Verification items for the finished model (mm, model axes). A direction names the side the tool comes from. Coordinates: 2 decimals unless noted, no trailing zeros. Order: outer loops, then holes, each group sorted by start corner. A loop starts at its lowest first (then second) coordinate and runs counter-clockwise, first axis right, second up. Notation, with made-up numbers: M -2,79 L 52,79 A32 ccw 52,109 Z; hole C 88,-1 d9. An arc over 180 degrees is marked long. Return JSON: item names as keys, results as strings.
Autodesk Inventor part; units mm, degrees
ref_plane "YZ Plane" through (0, 0, 0) normal (1, 0, 0) x (0, 1, 0)
ref_plane "XZ Plane" through (0, 0, 0) normal (0, 1, 0) x (-1, 0, 0)
ref_plane "XY Plane" through (0, 0, 0) normal (0, 0, 1) x (1, 0, 0)
sketch "Esquisse1" plane through (0, 0, 0) normal (0, 1, 0) x (-1, 0, 0)
  line L0 (28, -26) -> (-28, -26)
  line L1 (-28, -26) -> (-28, 26)
  line L2 (-28, 26) -> (28, 26)
  line L3 (28, 26) -> (28, -26)
  point P0 (0, 0)
  dimension "d0" = 56
  dimension "d1" = 28
  dimension "d2" = 52
  dimension "d3" = 26
extrude "Extrusion1" add sketch "Esquisse1" along normal blind 1.6
sketch "Esquisse2" plane through (0, 1.6, 0) normal (0, 1, 0) x (1, 0, 0)
  line L0 (-26, 24) -> (-23.5, 24)
  line L1 (-23.5, 24) -> (-23.5, -15)
  line L2 (-23.5, -15) -> (-26, -15)
  line L3 (-26, -15) -> (-26, 24)
  line L4 (22.5, 24) -> (25, 24)
  line L5 (25, 24) -> (25, -24)
  line L6 (25, -24) -> (22.5, -24)
  line L7 (22.5, -24) -> (22.5, 24)
  line L8 (28, 26) -> (-28, 26)
  line L9 (-28, 26) -> (-28, -26)
  point P0 (0, 0)
  dimension "d6" = 2.5
  dimension "d7" = 2.5
  dimension "d8" = 39
  dimension "d9" = 48
  dimension "d10" = 2
  dimension "d11" = 2
  dimension "d12" = 46
extrude "Extrusion2" add sketch "Esquisse2" along normal blind 3
properties part number "PCB Wifi" material "Nylon, disulfure de molybdène"
Q1. Draft check along X on faces 1 (the face through (-28, 1, 0)), 2 (the face through (22.5, 3, 0)), 3 (the face through (25, 3, 0)), 4 (the face through (-25, 3, 15)). Enter one of: pulls with the +X half, pulls with the -X half, needs draft (parallel to the pull), parting line crosses it, or undercut.
Values:
{"face 1": "pulls with the -X half", "face 2": "undercut", "face 3": "pulls with the +X half", "face 4": "needs draft"}
Q2. Tool access check on faces 5 (the face through (24, 3, -24)), 6 (the face through (24, 3, 24)), 7 (the face through (-23.5, 3, -5)), 8 (the face through (-26, 3, -4)). Record the directions out of +Z, -Z, +X, -X, +Y, -Y that give a thin tool (end or side, any length) a straight path to the whole face; none if there is none.
Values:
{"face 5": "-Z, +X, -X, +Y", "face 6": "+Z, +X, -X, +Y", "face 7": "+Z, -Z, +Y", "face 8": "+Z, -Z, -X, +Y"}
Q3. Cross-section at D-D, the plane z = -0.5. Record the boundary of the cut face in (x, y), and give its area (3 significant figures).
Values:
{"outline": "M -28,0 L 28,0 L 28,1.6 L 25,1.6 L 25,4.6 L 22.5,4.6 L 22.5,1.6 L -23.5,1.6 L -23.5,4.6 L -26,4.6 L -26,1.6 L -28,1.6 Z", "area": "105 mm^2"}
Q4. Material ranges on line 1 along X through (y, z) = (1.7, -4.5); line 2 along Y through (x, z) = (-6, -23); line 3 along X through (y, z) = (3.8, 15.5), recorded low to high.
Values:
{"line 1": "-26 to -23.5, 22.5 to 25", "line 2": "0 to 1.6", "line 3": "22.5 to 25"}
Q5. Cross-section at A-A, the plane y = 2.85. Record the boundary of the cut face in (x, z).
Values:
{"outline": "M -26,-24 L -23.5,-24 L -23.5,15 L -26,15 Z; M 22.5,-24 L 25,-24 L 25,24 L 22.5,24 Z"}
Q6. Cross-section at B-B, the plane z = 17.5. Record the boundary of the cut face in (x, y).
Values:
{"outline": "M -28,0 L 28,0 L 28,1.6 L 25,1.6 L 25,4.6 L 22.5,4.6 L 22.5,1.6 L -28,1.6 Z"}
Q7. Cross-section at C-C, the plane x = 3. Record the boundary of the cut face in (y, z).
Values:
{"outline": "M 0,-26 L 1.6,-26 L 1.6,26 L 0,26 Z"}
Q8. Go/stop test with flat-tipped pins: pin 1 (0.8 mm diameter, centred on x = 23, y = 4, fed in from -Z); pin 2 (2 mm diameter, centred on x = -24.5, y = 3, fed in from +Z); pin 3 (2 mm diameter, centred on x = 24, y = 3.5, fed in from +Z). Record where each tip stops, or that it passes through.
Values:
{"pin 1": "z = -24", "pin 2": "z = 15", "pin 3": "z = 24"}
